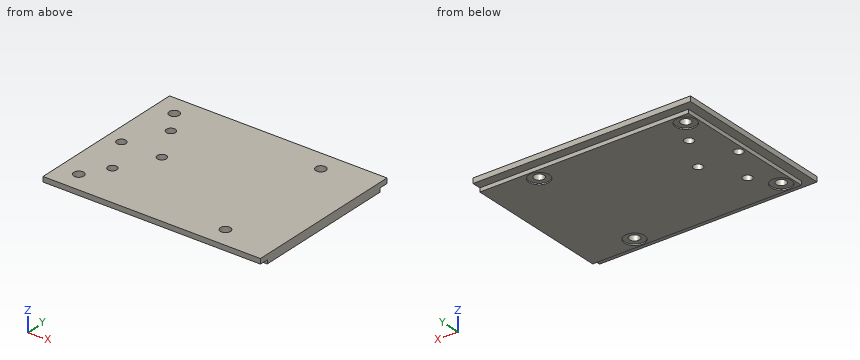
```python
from build123d import *

# Parameters (mm, degrees)
SKETCH1_W           = 82.5
SKETCH1_H           = 58
BOSS_EXTRUDE1_DEPTH = 1.5
SKETCH2_W           = 86
SKETCH2_H           = 65
BOSS_EXTRUDE2_DEPTH = 2
SKETCH3_R           = 2
CUT_EXTRUDE1_DEPTH  = 60.736923255
SKETCH4_R           = 1.8
CUT_EXTRUDE2_DEPTH  = 60.736923255
SKETCH5_R           = 4
CUT_EXTRUDE3_DEPTH  = 0.5


with BuildPart() as part:
    # Sketch1 → Boss-Extrude1 (new body)
    with BuildSketch(Plane.XY):
        with Locations((-5.25, 0)):
            Rectangle(SKETCH1_W, SKETCH1_H)
    extrude(amount=-BOSS_EXTRUDE1_DEPTH)

    # Sketch2 → Boss-Extrude2 (add)
    with BuildSketch(Plane.XY):
        with Locations((-7, 0)):
            Rectangle(SKETCH2_W, SKETCH2_H)
    extrude(amount=BOSS_EXTRUDE2_DEPTH)

    # Sketch3 → Cut-Extrude1 (cut, through all)
    with BuildSketch(Plane.XY.offset(2)):
        with Locations((-42, 24.5)):
            Circle(SKETCH3_R)
        with Locations((16, 24.5)):
            Circle(SKETCH3_R)
        with Locations((16, -24.5)):
            Circle(SKETCH3_R)
        with Locations((-42, -24.5)):
            Circle(SKETCH3_R)
    extrude(amount=-CUT_EXTRUDE1_DEPTH, mode=Mode.SUBTRACT)

    # Sketch4 → Cut-Extrude2 (cut, through all)
    with BuildSketch(Plane.XY.offset(2)):
        with Locations((-44, 0)):
            Circle(SKETCH4_R)
        with Locations((-28, 0)):
            Circle(SKETCH4_R)
        with Locations((-36, 15)):
            Circle(SKETCH4_R)
        with Locations((-36, -15)):
            Circle(SKETCH4_R)
    extrude(amount=-CUT_EXTRUDE2_DEPTH, mode=Mode.SUBTRACT)

    # Sketch5 → Cut-Extrude3 (cut)
    with BuildSketch(Plane(origin=(0, 0, -1.5), x_dir=(-1, 0, 0), z_dir=(0, 0, -1))):
        with Locations((-16, 24.5)):
            Circle(SKETCH5_R)
        with Locations((-16, -24.5)):
            Circle(SKETCH5_R)
        with Locations((42, -24.5)):
            Circle(SKETCH5_R)
        with Locations((42, 24.5)):
            Circle(SKETCH5_R)
    extrude(amount=-CUT_EXTRUDE3_DEPTH, mode=Mode.SUBTRACT)


solid = part.part
```
Geometry check sheet. Reference: the model listing, model coordinates, mm. Round coordinates to 2 decimals unless told otherwise and drop trailing zeros. Loops run counter-clockwise (first coordinate to the right, second up) from the corner with the lowest first, then second, coordinate; pieces in that order, holes last. Notation, with made-up numbers: M -28,-29 L 22,-29 A17 ccw 22,1 Z; hole C 85,2.25 d3. An arc over 180 degrees is marked long. Return JSON: item names as keys, results as strings. Group by question number.
(1) Scan lines: line 1 along Y through (x, z) = (-36, 0.8); line 2 along Y through (x, z) = (-42, -1.35); line 3 along Y through (x, z) = (-28, 0.2). Record each from-to range of solid material in increasing order. Write a range as [from, to].
(2) Section check D-D, the plane y = -24.5. Enter the section's corners in (x, z), and give its area (3 significant figures).
(3) Go/stop test with flat-tipped pins: pin 1 (0.8 mm diameter, centred on x = -20, z = -0.5, fed in from -Y); pin 2 (4 mm diameter, centred on x = -40.5, y = -24.5, fed in from -Z); pin 3 (0.8 mm diameter, centred on x = -9.5, z = -1, fed in from +Y). Record where each tip stops, or that it passes through.
(4) Section check B-B, the plane z = 1.05. Give the number of separate pieces and of enclosed holes in the cut face, and give its area (3 significant figures).
(5) Section check A-A, the plane x = -36. Enter the section's corners in (y, z).
(6) Section check C-C, the plane y = -15. Enter the section's corners in (x, z).
Data:
{
 "1": {"line 1": "[-32.5, -16.8], [-13.2, 13.2], [16.8, 32.5]", "line 2": "[-29, -28.5], [-20.5, 20.5], [28.5, 29]", "line 3": "[-32.5, -1.8], [1.8, 32.5]"},
 "2": {"outline": "M -50,0 L -46.5,0 L -46.5,-1.5 L -46,-1.5 L -46,-1 L -44,-1 L -44,2 L -50,2 Z; M -40,-1 L -38,-1 L -38,-1.5 L 12,-1.5 L 12,-1 L 14,-1 L 14,2 L -40,2 Z; M 18,-1 L 20,-1 L 20,-1.5 L 36,-1.5 L 36,2 L 18,2 Z", "area": "264 mm²"},
 "3": {"pin 1": "y = -29", "pin 2": "z = -1", "pin 3": "y = 29"},
 "4": {"separate pieces": "1", "enclosed holes": "8", "area": "5,500 mm²"},
 "5": {"outline": "M -32.5,0 L -29,0 L -29,-1.5 L -16.8,-1.5 L -16.8,2 L -32.5,2 Z; M -13.2,-1.5 L 13.2,-1.5 L 13.2,2 L -13.2,2 Z; M 16.8,-1.5 L 29,-1.5 L 29,0 L 32.5,0 L 32.5,2 L 16.8,2 Z"},
 "6": {"outline": "M -50,0 L -46.5,0 L -46.5,-1.5 L -37.8,-1.5 L -37.8,2 L -50,2 Z; M -34.2,-1.5 L 36,-1.5 L 36,2 L -34.2,2 Z"}
}
